The figure shows three views and two pictorial views of one solid part (mm, origin at its lowest corner). Answer the questions. Give positions to 0.01 mm unless a question says otherwise; leave off trailing zeros. Loops run counter-clockwise (first coordinate to the right, second up) from the corner with the lowest first, then second, coordinate; pieces in that order, holes last. Notation, with made-up numbers: (-39.75, -9) - (-3.75, -9) arc R32 cw to (-3.75, 22) - close; hole circle Ø7 at (84, 76). An arc over 180 degrees is marked (long way). One line per question, with ' | ' between items.
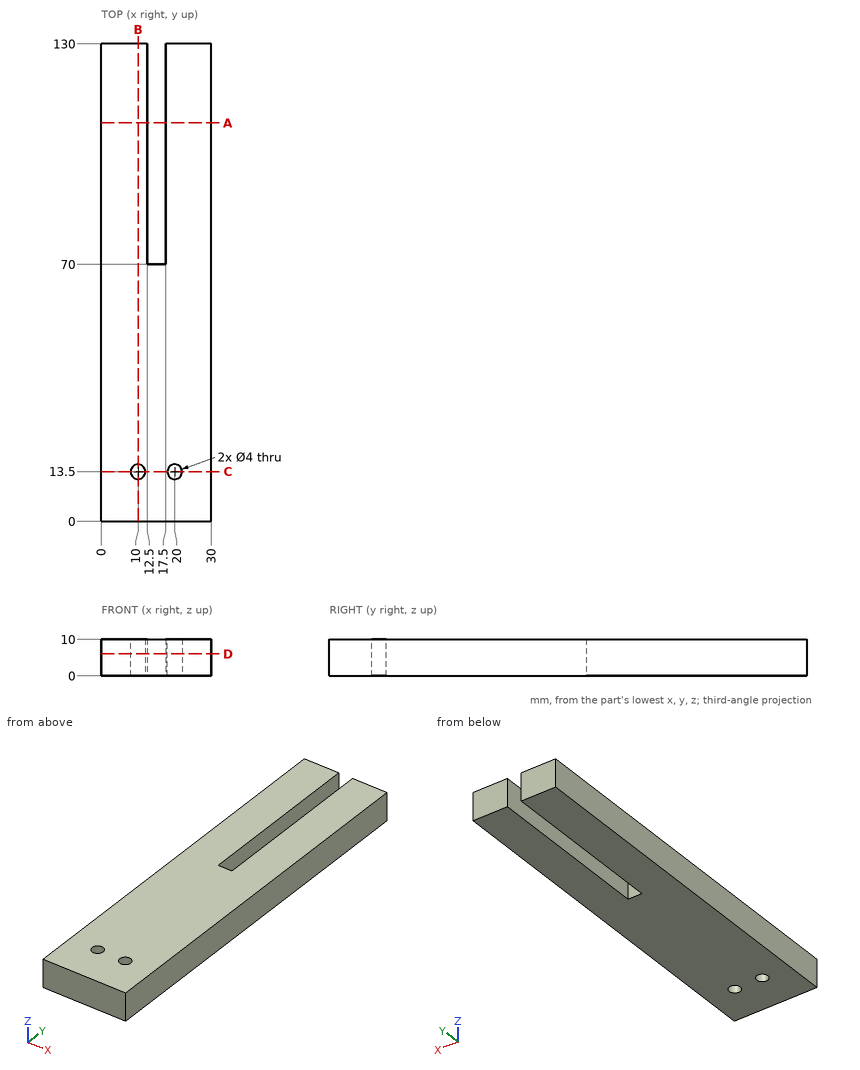
1. Consider L1, parallel to X at y = 99.5, z = 7; L2, parallel to Y at x = 20, z = 7.25. Determine where each line is inside the solid, lowest interval first.
Evaluation:
L1: 0 to 12.5, 17.5 to 30 | L2: 0 to 11.5, 15.5 to 130
2. Find section D-D on z = 6. Write down the section's boundary in (x, y), then the cut area to 3 significant figures.
Evaluation:
outline: (0, 0) - (30, 0) - (30, 130) - (17.5, 130) - (17.5, 70) - (12.5, 70) - (12.5, 130) - (0, 130) - close; hole circle Ø4 at (10, 13.5); hole circle Ø4 at (20, 13.5) | area: 3,570 mm2
3. Flat-ended cylindrical pins translate along their axes: pin 1 (6 mm diameter, centred on y = 89, z = 8.5, fed in from -X); pin 2 (1.5 mm diameter, centred on x = 15, z = 4, fed in from +Y). Find the tip coordinate at first contact, or state that the pin passes through.
Evaluation:
pin 1: x = 0 | pin 2: y = 70
4. Find section C-C on y = 13.5. Write down the section's boundary in (x, z), then the cut area to 3 significant figures.
Evaluation:
outline: (0, 0) - (8, 0) - (8, 10) - (0, 10) - close; (12, 0) - (18, 0) - (18, 10) - (12, 10) - close; (22, 0) - (30, 0) - (30, 10) - (22, 10) - close | area: 220 mm2
5. Find section A-A on y = 108.5. Write down the section's boundary in (x, z).
Evaluation:
outline: (0, 0) - (12.5, 0) - (12.5, 10) - (0, 10) - close; (17.5, 0) - (30, 0) - (30, 10) - (17.5, 10) - close
6. Find section B-B on x = 10. Write down the section's boundary in (y, z), then the cut area to 3 significant figures.
Evaluation:
outline: (0, 0) - (11.5, 0) - (11.5, 10) - (0, 10) - close; (15.5, 0) - (130, 0) - (130, 10) - (15.5, 10) - close | area: 1,260 mm2
